Design review of the part built by this model. Coordinates are the model's own, in mm. Face numbers are marked on the shaded views. A direction names the side the tool comes from. Give positions to 0.01 mm unless a question says otherwise; leave off trailing zeros. Order: outer loops, then holes, each group sorted by start corner. A loop starts at its lowest first (then second) coordinate and runs counter-clockwise, first axis right, second up.
```python
from build123d import *

# Parameters (mm, degrees)
CROQUIS2_R              = 1.45
SALIENTE_EXTRUIR1_DEPTH = 2.5
CROQUIS3_R              = 2.4
CROQUIS3_R_2            = 1.45
SALIENTE_EXTRUIR2_DEPTH = 3.5
CROQUIS4_R              = 1.575
CORTAR_EXTRUIR1_DEPTH   = 24.118782948


with BuildPart() as part:
    # Croquis2 → Saliente-Extruir1 (new body)
    with BuildSketch(Plane(origin=(0, 0, 0), x_dir=(1, 0, 0), z_dir=(0, 1, 0))):
        with BuildLine():
            Line((-3.45, 10), (-3.45, -10))
            ThreePointArc((-3.45, -10), (-1.630018545, -13.040647882), (1.909733068, -12.873224601))
            Line((1.909733068, -12.873224601), (16.923571713, -2.89404507))
            ThreePointArc((16.923571713, -2.89404507), (18.475, 0), (16.923571713, 2.89404507))
            Line((16.923571713, 2.89404507), (1.909733068, 12.873224601))
            ThreePointArc((1.909733068, 12.873224601), (-1.630018545, 13.040647882), (-3.45, 10))
        make_face()
        with Locations(Location((0, 10, 0), (0, 0, 270))):
            Circle(CROQUIS2_R, mode=Mode.SUBTRACT)
        with Locations(Location((0, -10, 0), (0, 0, 90))):
            Circle(CROQUIS2_R, mode=Mode.SUBTRACT)
    extrude(amount=SALIENTE_EXTRUIR1_DEPTH)

    # Croquis3 → Saliente-Extruir2 (add)
    # profile 1 of 2: a face of its own
    with BuildSketch(Plane(origin=(0, 2.5, 0), x_dir=(1, 0, 0), z_dir=(0, 1, 0))):
        with Locations(Location((0, 10, 0), (0, 0, 270))):
            Circle(CROQUIS3_R)
        with Locations(Location((0, 10, 0), (0, 0, 270))):
            Circle(CROQUIS3_R_2, mode=Mode.SUBTRACT)
    # profile 2 of 2: a face of its own
    with BuildSketch(Plane(origin=(0, 2.5, 0), x_dir=(1, 0, 0), z_dir=(0, 1, 0))):
        with Locations(Location((0, -10, 0), (0, 0, 270))):
            Circle(CROQUIS3_R)
        with Locations(Location((0, -10, 0), (0, 0, 90))):
            Circle(CROQUIS3_R_2, mode=Mode.SUBTRACT)
    extrude(amount=SALIENTE_EXTRUIR2_DEPTH)

    # Croquis4 → Cortar-Extruir1 (cut, through all)
    with BuildSketch(Plane(origin=(0, 2.5, 0), x_dir=(1, 0, 0), z_dir=(0, 1, 0))):
        with Locations(Location((15, 0, 0), (0, 0, 270))):
            Circle(CROQUIS4_R)
    extrude(amount=-CORTAR_EXTRUIR1_DEPTH, mode=Mode.SUBTRACT)


solid = part.part
```
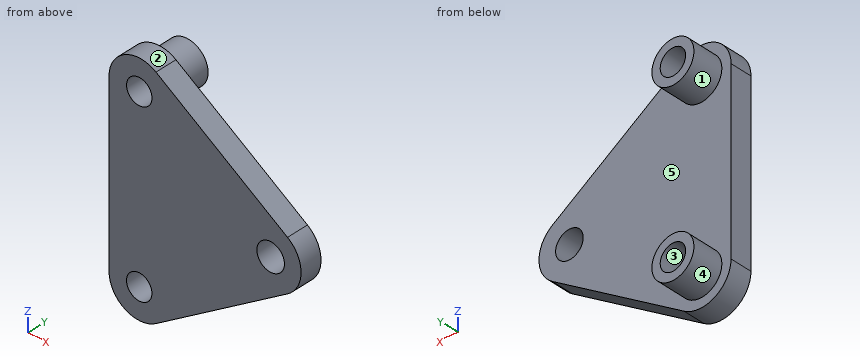
1. Take a section at B-B (y = 3.1). State the section outline as (x, z) points, then the cut area to 3 significant figures.
Recorded:
outline: circle Ø4.8 at (0, -10); circle Ø4.8 at (0, 10); hole circle Ø2.9 at (0, -10); hole circle Ø2.9 at (0, 10)
area: 23.0 mm2
2. Draft analysis for pull direction X (two halves, no side actions). For the marked faces 3, 4 and 5, state which applies: pulls with the +X half, pulls with the -X half, needs draft (parallel to the pull), parting line crosses it, or undercut.
Recorded:
face 3: undercut
face 4: parting line crosses it
face 5: needs draft
3. Take a section at A-A (x = 0). State the section outline as (y, z) points, then the cut area to 4 significant figures.
Recorded:
outline: (0, -13.45) - (2.5, -13.45) - (2.5, -12.4) - (6, -12.4) - (6, -11.45) - (0, -11.45) - close; (0, -8.55) - (6, -8.55) - (6, -7.6) - (2.5, -7.6) - (2.5, 7.6) - (6, 7.6) - (6, 8.55) - (0, 8.55) - close; (0, 11.45) - (6, 11.45) - (6, 12.4) - (2.5, 12.4) - (2.5, 13.45) - (0, 13.45) - close
area: 66.05 mm2
4. Machinability: for the marked faces 1 and 2, which of the approach directions +Z, -Z, +X, -X, +Y, -Y give a long, thin tool a straight path to every point of the face, cutting with its end or side? Answer none if there is none.
Recorded:
face 1: +Y
face 2: +Z, +Y, -Y
5. For pin 1 (1 mm diameter, centred on y = 1, z = -8.5, fed in from +X); pin 2 (2 mm diameter, centred on x = 5, y = 0.5, fed in from -Z); pin 3 (3 mm diameter, centred on x = 15, z = 0, fed in from +Y); pin 4 (3 mm diameter, centred on x = 0, y = 4.5, fed in from -Z), all flat-tipped, find the tip position at first contact; note any pin that passes through.
Recorded:
pin 1: stops at x = 9.24
pin 2: stops at z = -11.48
pin 3: passes through
pin 4: stops at z = -12.4
6. Take a section at D-D (x = 15). State the section outline as (y, z) points (3 decimals).
Recorded:
outline: (0, -4.173) - (2.5, -4.173) - (2.5, -1.575) - (0, -1.575) - close; (0, 1.575) - (2.5, 1.575) - (2.5, 4.173) - (0, 4.173) - close
7. Take a section at C-C (z = 0). State the section outline as (x, y) points (3 decimals).
Recorded:
outline: (-3.45, 0) - (13.425, 0) - (13.425, 2.5) - (-3.45, 2.5) - close; (16.575, 0) - (18.475, 0) - (18.475, 2.5) - (16.575, 2.5) - close
8. For line 1 along Y through (x, z) = (-0.25, -1); line 2 along Z through (x, y) = (1.25, 1.1); line 3 along X through (y, z) = (1.7, -8.75), list the stretches that pass through material, from the lowest coordinate up.
Recorded:
line 1: y = 0 to 2.5
line 2: z = -13.22 to -10.73, -9.27 to 9.27, 10.73 to 13.22
line 3: x = -3.45 to -0.73, 0.73 to 8.11
